from build123d import *

# Parameters (mm, degrees)
F1_DEPTH = 63.5
F0_W     = 25.4
F0_H     = 19.05
F0_H_2   = 4.7752
F0_H_3   = 4.7498
F2_DEPTH = 25.4
F4_DEPTH = 3.175
F5_R     = 12.7


with BuildPart() as f1:
    # F0 (on Front) → F1 (new body, symmetric)
    with BuildSketch(Plane.XZ):
        Polygon((-41.275, -9.525), (41.275, -9.525), (41.275, 9.525), (22.225, 9.525), (-41.275, 9.525), align=None)
    extrude(amount=F1_DEPTH, both=True)

    # F0 (on Front) → F2 (join, symmetric)
    with BuildSketch(Plane.XZ):
        with BuildLine():
            Line((22.225, 9.525), (41.275, 9.525))
            Line((41.275, 9.525), (41.275, 27.0002))
            ThreePointArc((41.275, 27.0002), (45.9246798487, 38.2255201513), (57.15, 42.8752))
            Line((57.15, 42.8752), (60.325, 42.8752))
            Line((60.325, 42.8752), (60.325, 61.9252))
            Line((60.325, 61.9252), (57.15, 61.9252))
            ThreePointArc((57.15, 61.9252), (32.4542956671, 51.6959043329), (22.225, 27.0002))
            Line((22.225, 27.0002), (22.225, 9.525))
        make_face()
        with Locations((73.025, 52.4002)):
            Rectangle(F0_W, F0_H)
        with Locations((73.025, 40.4876)):
            Rectangle(F0_W, F0_H_2)
        with Locations((73.025, 64.3001)):
            Rectangle(F0_W, F0_H_3)
    extrude(amount=F2_DEPTH, both=True)

    # F0 (on Front) → F3 (revolve)
    with BuildSketch(Plane.XZ):
        Polygon((85.725, 66.675), (85.725, 61.9252), (85.725, 42.8752), (85.725, 38.1), (111.125, 38.1), (111.125, 66.675), align=None)
    revolve(axis=Axis((85.725, 0, 52.3875), (0, 0, 1)))

    # F0 (on Front) → F4 (join, symmetric)
    with BuildSketch(Plane.XZ):
        with BuildLine():
            add(Edge.make_bspline(
                [(-41.275, 9.525), (-42.3543564975, 56.6976591945), (4.171225708, 62.171254307), (57.15, 61.9252)],
                knots=[0, 0, 0, 0, 111.5045361635, 111.5045361635, 111.5045361635, 111.5045361635], degree=3))
            Line((-41.275, 9.525), (22.225, 9.525))
            Line((22.225, 9.525), (22.225, 27.0002))
            ThreePointArc((22.225, 27.0002), (32.4542956671, 51.6959043329), (57.15, 61.9252))
        make_face()
    extrude(amount=F4_DEPTH, both=True)

    # F5
    f5_edges = [f1.edges().sort_by_distance(p)[0] for p in [
        (85.725, 25.4, 52.3875),
        (73.025, 25.4, 66.675),
        (73.025, -25.4, 66.675),
        (111.125, 0, 66.675),
    ]]
    fillet(f5_edges, radius=F5_R)


solid = f1.part
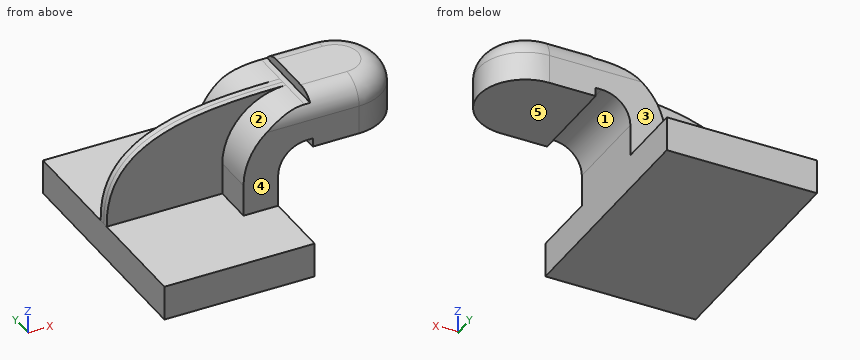
The model under review builds one solid part; all positions refer to its coordinate system, in mm. Face numbers are marked on the shaded views. A direction names the side the tool comes from. Round coordinates to 2 decimals unless told otherwise and drop trailing zeros. Write each loop counter-clockwise with the first axis right and the second up, starting at its lowest first coordinate (ties: lowest second). Pieces come first, ordered by that corner, then holes. Notation, with made-up numbers: M 59.5,-8.75 L 72.5,-8.75 A26 cw 72.5,27.25 Z; hole C -24.5,82.5 d9. An arc over 180 degrees is marked long. Use a Markdown table: item, result. Add a question column.
Q1. We need section B-B, the plane y = 41.5. State the section outline as (x, z) points (3 decimals).
Q2. We need section A-A, the plane z = 5.5. State the section outline as (x, y) points (3 decimals), plus the area to 3 significant figures.
Q3. To check wall thickness, follow line 1 (X direction, y = 19.5, z = 14.5) (3 decimals); line 2 (Z direction, x = 21, y = 52.5) (3 decimals); line 3 (X direction, y = -50, z = -5) (3 decimals). State the ranges of each line that lie inside material, in increasing order.
Q4. Insertion check: pin 1 (5.5 mm diameter, centred on y = -14, z = 1, fed in from -X) (3 decimals); pin 2 (14 mm diameter, centred on y = 12.5, z = 20.5, fed in from -X) (3 decimals); pin 3 (4 mm diameter, centred on y = -3, z = -1, fed in from +X) (3 decimals). Each pin has a flat end and moves straight along its axis. Give the tip position at first contact, or say it passes through.
Q5. Machinability: for the marked faces 1, 2, 3, 4 and 5, which of the approach directions +Z, -Z, +X, -X, +Y, -Y give a long, thin tool a straight path to every point of the face, cutting with its end or side? Answer none if there is none.
Findings below:
| question | item | result |
|---|---|---|
| 1 | outline | M -41.275,-9.525 L 41.275,-9.525 L 41.275,9.525 L -41.275,9.525 Z |
| 2 | outline | M -41.275,-63.5 L 41.275,-63.5 L 41.275,63.5 L -41.275,63.5 Z |
| 2 | area | 10,500 mm² |
| 3 | line 1 | x = 22.225 to 41.275 |
| 3 | line 2 | z = -9.525 to 9.525 |
| 3 | line 3 | x = -41.275 to 41.275 |
| 4 | pin 1 | stops at x = -41.275 |
| 4 | pin 2 | stops at x = 22.225 |
| 4 | pin 3 | stops at x = 41.275 |
| 5 | face 1 | -Z, +Y, -Y |
| 5 | face 2 | +Z, -X, -Y |
| 5 | face 3 | +Z, +X, -X, +Y |
| 5 | face 4 | +Z, +X, -X, -Y |
| 5 | face 5 | -Z, +X, +Y, -Y |
